The drawing under review shows one solid part. Ordinate dimensions are in mm from its lowest x, y, z. Coordinates: 2 decimals unless noted, no trailing zeros. Write each loop counter-clockwise with the first axis right and the second up, starting at its lowest first coordinate (ties: lowest second). Pieces come first, ordered by that corner, then holes. Notation, with made-up numbers: M 70.25,32.25 L 128.25,32.25 A22 cw 128.25,38.25 Z; hole C 15,26 d6. An arc over 180 degrees is marked long. Write item = value, one per line.
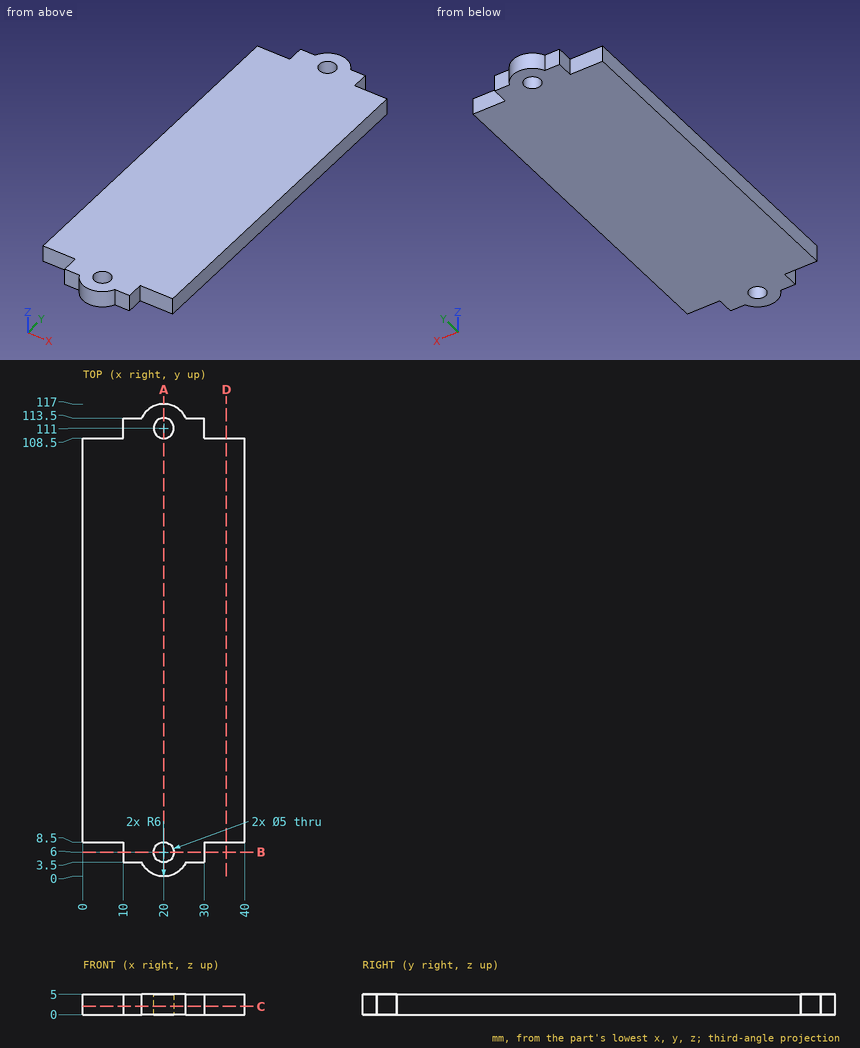
Q1. Consider section C-C, the plane z = 2.05. State the section outline as (x, y) points, and give its area (3 significant figures).
Check result:
outline = M 0,8.5 L 10,8.5 L 10,3.5 L 14.55,3.5 A6 ccw 25.45,3.5 L 30,3.5 L 30,8.5 L 40,8.5 L 40,108.5 L 30,108.5 L 30,113.5 L 25.45,113.5 A6 ccw 14.55,113.5 L 10,113.5 L 10,108.5 L 0,108.5 Z; hole C 20,6 d5; hole C 20,111 d5
area = 4,220 mm²
Q2. Wall thickness on line 1 (Y direction, x = 20, z = 1); line 2 (X direction, y = 6, z = 1.8); line 3 (Y direction, x = 22, z = 2.15): over which ranges is each line inside the solid? List them lowest first.
Check result:
line_1 = 0 to 3.5, 8.5 to 108.5, 113.5 to 117
line_2 = 10 to 17.5, 22.5 to 30
line_3 = 0.34 to 4.5, 7.5 to 109.5, 112.5 to 116.66
Q3. For P1, Ø2, axis at x = 19, z = 2.5, coming from the -Y side; P2, Ø2.5, axis at y = 110, z = 2.5, coming from the +X side; P3, Ø1.5, axis at x = 14, z = 1, coming from the -Y side; P4, Ø2.5, axis at x = 13, z = 2.5, coming from the -Y side, all flat-tipped, find the tip position at first contact; note any pin that passes through.
Check result:
P1 = 0
P2 = 30
P3 = 3.1
P4 = 3.5
Q4. Consider section A-A, the plane x = 20. State the section outline as (y, z) points.
Check result:
outline = M 0,0 L 3.5,0 L 3.5,5 L 0,5 Z; M 8.5,0 L 108.5,0 L 108.5,5 L 8.5,5 Z; M 113.5,0 L 117,0 L 117,5 L 113.5,5 Z
Q5. Consider section D-D, the plane x = 35.5. State the section outline as (y, z) points, and give its area (3 significant figures).
Check result:
outline = M 8.5,0 L 108.5,0 L 108.5,5 L 8.5,5 Z
area = 500 mm²
Q6. Consider section B-B, the plane y = 6. State the section outline as (x, z) points, and give its area (3 significant figures).
Check result:
outline = M 10,0 L 17.5,0 L 17.5,5 L 10,5 Z; M 22.5,0 L 30,0 L 30,5 L 22.5,5 Z
area = 75.0 mm²
